from build123d import *

# Parameters (mm, degrees)
SKETCH_1_W               = 60
SKETCH_1_H               = 26
EXTRUDE_1_DEPTH          = 24
CUT_EXTRUDE_1_DEPTH      = 1
CUT_EXTRUDE_1_DEPTH_BACK = 24
SKETCH_3_W               = 23
SKETCH_3_H               = 24
EXTRUDE_2_DEPTH          = 10
CUT_EXTRUDE_2_DEPTH      = 25
SKETCH_5_W               = 23
SKETCH_5_H               = 1
CUT_EXTRUDE_3_DEPTH      = 25
SKETCH_6_W               = 24.56
SKETCH_6_H               = 24
EXTRUDE_4_DEPTH          = 15.5
CUT_EXTRUDE_5_DEPTH      = 4
CUT_EXTRUDE_6_DEPTH      = 11
SKETCH_10_W              = 8
SKETCH_10_H              = 0.5
CUT_EXTRUDE_8_DEPTH      = 25
SKETCH_11_R              = 1
CUT_EXTRUDE_9_DEPTH      = 11
SKETCH_12_W              = 24
SKETCH_12_H              = 4
EXTRUDE_5_DEPTH          = 20
SKETCH_13_W              = 24
SKETCH_13_H              = 4
EXTRUDE_6_DEPTH          = 20
CUT_EXTRUDE_10_DEPTH     = 4
FILLET_1_R               = 1
SKETCH_15_R              = 2.6
CUT_EXTRUDE_11_DEPTH     = 4
SKETCH_16_R              = 2.6
CUT_EXTRUDE_12_DEPTH     = 4
SKETCH_17_W              = 20
SKETCH_17_H              = 22
CUT_EXTRUDE_13_DEPTH     = 0.1
SKETCH_18_W              = 20
SKETCH_18_H              = 10.5
CUT_EXTRUDE_14_DEPTH     = 0.1


with BuildPart() as part:
    # 草图1 → 凸台-拉伸1 (new body)
    with BuildSketch(Plane.XY):
        with Locations((5.238297872, -1.05106383)):
            Rectangle(SKETCH_1_W, SKETCH_1_H)
    extrude(amount=-EXTRUDE_1_DEPTH)

    # 草图2 → 切除-拉伸1 (cut, two sides)
    with BuildSketch(Plane.XY) as cut_extrude_1_sk:
        Polygon((-20.761702128, 145.431728494), (-20.761702128, 11.94893617), (-20.761702128, -10.05106383), (31.238297872, -10.05106383), (31.238297872, 11.94893617), (31.238297872, 145.431728494), (31.238297872, 412.397313141), (-20.761702128, 412.397313141), align=None)
    extrude(amount=CUT_EXTRUDE_1_DEPTH, mode=Mode.SUBTRACT)
    extrude(cut_extrude_1_sk.sketch, amount=-CUT_EXTRUDE_1_DEPTH_BACK, mode=Mode.SUBTRACT)

    # 草图3 → 凸台-拉伸2 (add)
    with BuildSketch(Plane(origin=(0, -10.05106383, 0), x_dir=(1, 0, 0), z_dir=(0, 1, 0))):
        with Locations((15.298297872, 12)):
            Rectangle(SKETCH_3_W, SKETCH_3_H)
    extrude(amount=EXTRUDE_2_DEPTH)

    # 草图4 → 切除-拉伸2 (cut, through all)
    with BuildSketch(Plane.XY):
        with BuildLine():
            Line((7.798297872, -0.05106383), (22.798297872, -0.05106383))
            ThreePointArc((22.798297872, -0.05106383), (15.298297872, -7.55106383), (7.798297872, -0.05106383))
        make_face()
    extrude(amount=-CUT_EXTRUDE_2_DEPTH, mode=Mode.SUBTRACT)

    # 草图5 → 切除-拉伸3 (cut, through all)
    with BuildSketch(Plane.XY):
        with Locations((15.298297872, -0.55106383)):
            Rectangle(SKETCH_5_W, SKETCH_5_H)
    extrude(amount=-CUT_EXTRUDE_3_DEPTH, mode=Mode.SUBTRACT)

    # 草图6 → 凸台-拉伸4 (add)
    with BuildSketch(Plane(origin=(0, -10.05106383, 0), x_dir=(1, 0, 0), z_dir=(0, 1, 0))):
        with Locations((-8.481702128, 12)):
            Rectangle(SKETCH_6_W, SKETCH_6_H)
    extrude(amount=EXTRUDE_4_DEPTH)

    # 草图7 → 切除-拉伸5 (cut)
    with BuildSketch(Plane(origin=(0, 5.44893617, 0), x_dir=(1, 0, 0), z_dir=(0, 1, 0))):
        Polygon((-20.761702128, 0), (-11.241702128, 0), (-11.241702128, 12), (-3.241702128, 12), (-3.241702128, 0), (3.798297872, 0), (3.798297872, 24), (-20.761702128, 24), align=None)
    extrude(amount=-CUT_EXTRUDE_5_DEPTH, mode=Mode.SUBTRACT)

    # 草图8 → 切除-拉伸6 (cut)
    with BuildSketch(Plane.XY):
        with BuildLine():
            Line((-9.241702128, 5.44893617), (-5.241702128, 5.44893617))
            ThreePointArc((-5.241702128, 5.44893617), (-7.241702128, 3.44893617), (-9.241702128, 5.44893617))
        make_face()
    extrude(amount=-CUT_EXTRUDE_6_DEPTH, mode=Mode.SUBTRACT)

    # 草图10 → 切除-拉伸8 (cut, through all)
    with BuildSketch(Plane.XY):
        with Locations((-7.241702128, 5.19893617)):
            Rectangle(SKETCH_10_W, SKETCH_10_H)
    extrude(amount=-CUT_EXTRUDE_8_DEPTH, mode=Mode.SUBTRACT)

    # 草图11 → 切除-拉伸9 (cut)
    with BuildSketch(Plane(origin=(0, 0, -12), x_dir=(-1, 0, 0), z_dir=(0, 0, -1))):
        with Locations((7.241702128, 4.94893617)):
            Circle(SKETCH_11_R)
    extrude(amount=-CUT_EXTRUDE_9_DEPTH, mode=Mode.SUBTRACT)

    # 草图12 → 凸台-拉伸5 (add)
    with BuildSketch(Plane(origin=(35.238297872, 0, 0), x_dir=(0, 0, -1), z_dir=(1, 0, 0))):
        with Locations((12, 9.94893617)):
            Rectangle(SKETCH_12_W, SKETCH_12_H)
    extrude(amount=EXTRUDE_5_DEPTH)

    # 草图13 → 凸台-拉伸6 (add)
    with BuildSketch(Plane.ZY.offset(24.761702128)):
        with Locations((-12, 9.94893617)):
            Rectangle(SKETCH_13_W, SKETCH_13_H)
    extrude(amount=EXTRUDE_6_DEPTH)

    # 草图14 → 切除-拉伸10 (cut)
    with BuildSketch(Plane.XY):
        with BuildLine():
            Line((-9.178193801, 4.94893617), (-11.241702128, 4.94893617))
            Line((-11.241702128, 4.94893617), (-11.241702128, 1.44893617))
            Line((-11.241702128, 1.44893617), (-20.761702128, 1.44893617))
            Line((-20.761702128, 1.44893617), (-20.761702128, 11.94893617))
            Line((-20.761702128, 11.94893617), (-44.761702128, 11.94893617))
            Line((-44.761702128, 11.94893617), (-44.761702128, 7.94893617))
            Line((-44.761702128, 7.94893617), (-24.761702128, 7.94893617))
            Line((-24.761702128, 7.94893617), (-24.761702128, -14.05106383))
            Line((-24.761702128, -14.05106383), (35.238297872, -14.05106383))
            Line((35.238297872, -14.05106383), (35.238297872, 7.94893617))
            Line((35.238297872, 7.94893617), (55.238297872, 7.94893617))
            Line((55.238297872, 7.94893617), (55.238297872, 11.94893617))
            Line((55.238297872, 11.94893617), (31.238297872, 11.94893617))
            Line((31.238297872, 11.94893617), (31.238297872, -10.05106383))
            Line((31.238297872, -10.05106383), (26.798297872, -10.05106383))
            Line((26.798297872, -10.05106383), (26.798297872, -1.05106383))
            Line((26.798297872, -1.05106383), (22.731332246, -1.05106383))
            ThreePointArc((22.731332246, -1.05106383), (15.298297872, -7.55106383), (7.865263499, -1.05106383))
            Line((7.865263499, -1.05106383), (3.798297872, -1.05106383))
            Line((3.798297872, -1.05106383), (3.798297872, 1.44893617))
            Line((3.798297872, 1.44893617), (-3.241702128, 1.44893617))
            Line((-3.241702128, 1.44893617), (-3.241702128, 4.94893617))
            Line((-3.241702128, 4.94893617), (-5.305210455, 4.94893617))
            ThreePointArc((-5.305210455, 4.94893617), (-7.241702128, 3.44893617), (-9.178193801, 4.94893617))
        make_face()
    extrude(amount=-CUT_EXTRUDE_10_DEPTH, mode=Mode.SUBTRACT)

    # 圆角1
    fillet_1_edges = [part.edges().sort_by_distance(p)[0] for p in [
        (35.238297872, -3.05106383, -24),
        (45.238297872, 7.94893617, -24),
        (-24.761702128, -3.05106383, -24),
        (-34.761702128, 7.94893617, -24),
        (-44.761702128, 7.94893617, -14),
        (55.238297872, 7.94893617, -14),
        (45.238297872, 7.94893617, -4),
        (35.238297872, -3.05106383, -4),
        (5.238297872, -14.05106383, -4),
        (-24.761702128, -3.05106383, -4),
        (-34.761702128, 7.94893617, -4),
        (35.238297872, -14.05106383, -14),
        (-24.761702128, -14.05106383, -14),
        (5.238297872, -14.05106383, -24),
    ]]
    fillet(fillet_1_edges, radius=FILLET_1_R)

    # 草图15 → 切除-拉伸11 (cut)
    with BuildSketch(Plane(origin=(0, 7.94893617, 0), x_dir=(-1, 0, 0), z_dir=(0, -1, 0))):
        with Locations((34.261702128, 14)):
            Circle(SKETCH_15_R)
    extrude(amount=-CUT_EXTRUDE_11_DEPTH, mode=Mode.SUBTRACT)

    # 草图16 → 切除-拉伸12 (cut)
    with BuildSketch(Plane(origin=(0, 7.94893617, 0), x_dir=(-1, 0, 0), z_dir=(0, -1, 0))):
        with Locations((-44.738297872, 14)):
            Circle(SKETCH_16_R)
    extrude(amount=-CUT_EXTRUDE_12_DEPTH, mode=Mode.SUBTRACT)

    # 草图17 → 切除-拉伸13 (cut)
    with BuildSketch(Plane.ZY.offset(-31.238297872)):
        with Locations((-14, 0.94893617)):
            Rectangle(SKETCH_17_W, SKETCH_17_H)
    extrude(amount=-CUT_EXTRUDE_13_DEPTH, mode=Mode.SUBTRACT)

    # 草图18 → 切除-拉伸14 (cut)
    with BuildSketch(Plane(origin=(-20.761702128, 0, 0), x_dir=(0, 0, -1), z_dir=(1, 0, 0))):
        with Locations((14, 6.69893617)):
            Rectangle(SKETCH_18_W, SKETCH_18_H)
    extrude(amount=-CUT_EXTRUDE_14_DEPTH, mode=Mode.SUBTRACT)


solid = part.part
Can you work these out from the model? Positions are in its coordinate system, mm. A direction names the side the tool comes from. Round coordinates to 2 decimals unless told otherwise and drop trailing zeros. Write each loop counter-clockwise with the first axis right and the second up, starting at its lowest first coordinate (ties: lowest second). Pieces come first, ordered by that corner, then holes. Notation, with made-up numbers: M 20,-26 L 35,-26 A6 cw 35,-20 Z; hole C 77,57 d6. An arc over 180 degrees is marked long. Use CSV: the item, a comma, the result in double quotes.
(1) I'm going to push flat-ended pins straight in: pin 1 (10 mm diameter, centred on y = -3.5, z = -10.5, fed in from +X); pin 2 (1 mm diameter, centred on x = -6, y = 4, fed in from -Z); pin 3 (5 mm diameter, centred on x = -24, y = 3.5, fed in from -Z); pin 4 (3.5 mm diameter, centred on x = 29, z = -10.5, fed in from +Y). Where does each tip first touch, or does it pass through?
Check values:
pin 1,"x = 35.24"
pin 2,"z = -12"
pin 3,"z = -24"
pin 4,"y = -10.05"
(2) Imagine slicing it at D-D (x = -39). Write out the boundary of the cut face in (y, z).
Check values:
outline,"M 7.95,-23 A1 ccw 8.95,-24 L 11.95,-24 L 11.95,-4 L 8.95,-4 A1 ccw 7.95,-5 Z"
(3) Imagine slicing it at A-A (z = -14). Count the separate pieces of the cut face and the enclosed holes in it, plus the area to 3 significant figures.
Check values:
separate pieces,"3"
enclosed holes,"0"
area,"946 mm^2"
(4) Imagine slicing it at C-C (y = -2.75). Write out the boundary of the cut face in (x, z).
Check values:
outline,"M -24.76,-23 A1 ccw -23.76,-24 L 8.3,-24 L 8.3,-4 L -23.76,-4 A1 ccw -24.76,-5 Z; M 22.3,-24 L 26.8,-24 L 26.8,-4 L 22.3,-4 Z; M 31.34,-24 L 34.24,-24 A1 ccw 35.24,-23 L 35.24,-5 A1 ccw 34.24,-4 L 31.34,-4 Z"
(5) Imagine slicing it at B-B (z = -7.5). Write out the boundary of the cut face in (x, y), plus the area to 3 significant figures.
Check values:
outline,"M -44.76,8.95 A1 ccw -43.76,7.95 L -24.76,7.95 L -24.76,-13.05 A1 ccw -23.76,-14.05 L 34.24,-14.05 A1 ccw 35.24,-13.05 L 35.24,7.95 L 54.24,7.95 A1 ccw 55.24,8.95 L 55.24,11.95 L 31.34,11.95 L 31.34,-10.05 L 26.8,-10.05 L 26.8,-1.05 L 22.73,-1.05 A7.5 cw 7.87,-1.05 L 3.8,-1.05 L 3.8,1.45 L -3.24,1.45 L -3.24,4.95 L -5.31,4.95 A2 cw -9.18,4.95 L -11.24,4.95 L -11.24,1.45 L -20.86,1.45 L -20.86,11.95 L -44.76,11.95 Z"
area,"1,010 mm^2"
(6) I need wall thicknesses on line 1 along X through (y, z) = (9, -14); line 2 along X through (y, z) = (0.75, -8.25); line 3 along X through (y, z) = (4.25, -20.5). Which ranges of each line are inside material? Lowest first, please.
Check values:
line 1,"-44.76 to -36.86, -31.66 to -20.86, 31.34 to 42.14, 47.34 to 55.24"
line 2,"-24.76 to 3.8, 31.34 to 35.24"
line 3,"-24.76 to -20.86, 31.34 to 35.24"
(7) On a 3-axis mill with a long thin cutter (end or side, diameter ignored), from which of +Z, -Z, +X, -X, +Y, -Y can I reach the whole of each face in a straight line? I mean faces 1 (the flat face through (42, 7.949, -16)), 2 (the flat face through (3.798, 0, -14)), 3 (the flat face through (-2, -3, -4)), 4 (the flat face through (-32, 7.949, -12)). Say none if no direction works.
Check values:
face 1,"+Z, -Z, +X, -Y"
face 2,"+Z, -Z, +Y"
face 3,"+Z, +X, -X, +Y, -Y"
face 4,"+Z, -Z, -X, -Y"
(8) We'd pull the mould along Z, two halves only. Please class faces 5 (the flat face through (55.238, 10, -14)), 6 (the flat face through (-7, 3, -12)), 7 (the cylindrical face through (42.26, 9.92, -14.78)): +Z half, -Z half, draft (parallel to the pull), parting line (faces both ways), or undercut.
Check values:
face 5,"draft"
face 6,"-Z half"
face 7,"undercut"
